Geometry check sheet. Reference: the model listing, model coordinates, mm. A direction names the side the tool comes from. Round coordinates to 2 decimals unless told otherwise and drop trailing zeros. Write each loop counter-clockwise with the first axis right and the second up, starting at its lowest first coordinate (ties: lowest second). Pieces come first, ordered by that corner, then holes.
Item 1: Cross-section at C-C (z = 4.5). Enter the section's corners in (x, y).
Item 2: Cross-section at D-D (x = -0.25). Enter the section's corners in (y, z), then the cut area to 3 significant figures.
Item 3: Depth check by flat-ended pin: P1, Ø0.6, axis at x = 5, z = 1.5, coming from the -Y side; P2, Ø0.8, axis at y = 0.5, z = -3, coming from the +X side; P3, Ø3.5, axis at x = 10.1, z = -1.5, coming from the +Y side. Enter the tip coordinate at first touch or a pass-through.
Item 4: Draft check along Y on faces 1 (the face through (2.2, 4.2, 3.5)), 2 (the face through (5.754, -5.325, 1.728)), 3 (the face through (10, 3.5, 2)), 4 (the face through (4.5, 2.6, 0.8)). Enter one of: pulls with the +Y half, pulls with the -Y half, needs draft (parallel to the pull), parting line crosses it, or undercut.
Item 5: Cross-section at A-A (z = -1.5). Enter the section's corners in (x, y), then the cut area to 3 significant figures.
Item 6: Cross-section at B-B (z = 10.25). Enter the section's corners in (x, y).
Item 7: Access from +Z, -Z, +X, -X, +Y, -Y to the whole of each face (thin tool, end or side, straight path). Record for faces 5 (the face through (0, 0, 0)), 6 (the face through (6.81, 4.49, -0.13)), 7 (the face through (7.6, 3, 0)), 8 (the face through (10, 4, 2)), 9 (the face through (-4, 1, 3.5)).
Item 8: Scan lines: probe 1 along X at (y, z) = (3.75, -1.5); probe 2 along X at (y, z) = (3.95, 4.5); probe 3 along Y at (x, z) = (5.8, 1.5). Record each from-to range of solid material in increasing order.
from build123d import *

# Parameters (mm, degrees)
SKETCH1_W            = 9
SKETCH1_H            = 7
BOSS_EXTRUDE1_DEPTH  = 7
SKETCH4_W            = 0.725
SKETCH4_H            = 0.725
BOSS_EXTRUDE3_DEPTH  = 0.3
SKETCH7_W            = 6.8
SKETCH7_H            = 1
BOSS_EXTRUDE5_DEPTH  = 1
FILLET1_R            = 0.5
SKETCH8_W            = 15.5
SKETCH8_H            = 14
BOSS_EXTRUDE6_DEPTH  = 0.5
EXTRUDE_9_DEPTH      = 10
EXTRUDE_9_DEPTH_BACK = 2.1
SKETCH_6_R           = 1
SKETCH10_W           = 10.53
SKETCH10_H           = 0.5
BOSS_EXTRUDE9_DEPTH  = 5
SKETCH_3_R           = 1.05
CUT_EXTRUDE_2_DEPTH  = 0.5
SKETCH_5_R           = 3.25
EXTRUDE_2_DEPTH      = 20.5
SKETCH_7_R           = 1.05
CUT_EXTRUDE_3_DEPTH  = 1.6


with BuildPart() as part:
    # Sketch1 → Boss-Extrude1 (new body)
    with BuildSketch(Plane(origin=(0, 0, 0), x_dir=(1, 0, 0), z_dir=(0, 1, 0))):
        Rectangle(SKETCH1_W, SKETCH1_H)
    extrude(amount=BOSS_EXTRUDE1_DEPTH)

    # Sketch4 → Boss-Extrude3 (add)
    with BuildSketch(Plane(origin=(4.5, 0, 0), x_dir=(0, 0, -1), z_dir=(1, 0, 0))):
        with Locations((-3.1375, 6.6375)):
            Rectangle(SKETCH4_W, SKETCH4_H)
        with Locations((3.1375, 6.6375)):
            Rectangle(SKETCH4_W, SKETCH4_H)
        with Locations((-3.1375, 0.3625)):
            Rectangle(SKETCH4_W, SKETCH4_H)
        with Locations((3.1375, 0.3625)):
            Rectangle(SKETCH4_W, SKETCH4_H)
    extrude(amount=BOSS_EXTRUDE3_DEPTH)

    # Sketch7 → Boss-Extrude5 (add)
    with BuildSketch(Plane(origin=(4.5, 0, 0), x_dir=(0, 0, -1), z_dir=(1, 0, 0))):
        with Locations((0, 0.6)):
            Rectangle(SKETCH7_W, SKETCH7_H)
        with Locations((0, 6.4)):
            Rectangle(SKETCH7_W, SKETCH7_H)
    extrude(amount=BOSS_EXTRUDE5_DEPTH)

    # Fillet1
    # the kernel refuses this fillet: 0.5 mm, written as the material it adds along each edge
    with BuildSketch(Plane(origin=(4.5, 6.9, 3.525), x_dir=(0, 1, 0), z_dir=(0, 0, -1))) as fillet1_piece_1_section:
        with BuildLine():
            CenterArc((0.5, 0.3), FILLET1_R, 180, 36.869897646)
            Line((0, 0.3), (0, 0))
            Line((0, 0), (0.1, 0))
        make_face()
    fillet1_piece_1 = extrude(amount=7.05, mode=Mode.PRIVATE)
    fillet1_piece_1 = split(fillet1_piece_1, bisect_by=Plane(origin=(4.5, 6.9, -3.4), z_dir=(0, 0, 1)), keep=Keep.TOP, mode=Mode.PRIVATE)
    fillet1_piece_1 = split(fillet1_piece_1, bisect_by=Plane(origin=(4.5, 6.9, 3.4), z_dir=(0, 0, -1)), keep=Keep.TOP, mode=Mode.PRIVATE)
    add(fillet1_piece_1)
    with BuildSketch(Plane(origin=(4.5, 5.9, 3.4), x_dir=(0, 0, 1), z_dir=(0, 1, 0))) as fillet1_piece_2:
        with BuildLine():
            CenterArc((0.5, 0.3), FILLET1_R, 180, 36.869897646)
            Line((0, 0.3), (0, 0))
            Line((0, 0), (0.1, 0))
        make_face()
    extrude(amount=0.375)
    with BuildSketch(Plane(origin=(4.5, 5.9, -3.4), x_dir=(0, -1, 0), z_dir=(0, 0, 1)), Plane(origin=(4.5, 1.1, 3.4), x_dir=(0, 1, 0), z_dir=(0, 0, -1))) as fillet1_piece_3:
        with BuildLine():
            CenterArc((FILLET1_R, FILLET1_R), FILLET1_R, 180, 90)
            Line((0, FILLET1_R), (0, 0))
            Line((0, 0), (FILLET1_R, 0))
        make_face()
    extrude(amount=6.8)
    with BuildSketch(Plane(origin=(4.5, 7.025, -3.4), x_dir=(0, 0, -1), z_dir=(0, -1, 0))) as fillet1_piece_4_section:
        with BuildLine():
            CenterArc((0.5, 0.3), FILLET1_R, 180, 36.869897646)
            Line((0, 0.3), (0, 0))
            Line((0, 0), (0.1, 0))
        make_face()
    fillet1_piece_4 = extrude(amount=1.125, mode=Mode.PRIVATE)
    fillet1_piece_4 = split(fillet1_piece_4, bisect_by=Plane(origin=(4.5, 6.9, -3.4), z_dir=(0, -1, 0)), keep=Keep.TOP, mode=Mode.PRIVATE)
    add(fillet1_piece_4)
    with BuildSketch(Plane(origin=(4.5, 1.1, -3.4), x_dir=(0, 0, -1), z_dir=(0, -1, 0))) as fillet1_piece_5_section:
        with BuildLine():
            CenterArc((0.5, 0.3), FILLET1_R, 180, 36.869897646)
            Line((0, 0.3), (0, 0))
            Line((0, 0), (0.1, 0))
        make_face()
    fillet1_piece_5 = extrude(amount=1.125, mode=Mode.PRIVATE)
    fillet1_piece_5 = split(fillet1_piece_5, bisect_by=Plane(origin=(4.5, 0.1, -3.4), z_dir=(0, 1, 0)), keep=Keep.TOP, mode=Mode.PRIVATE)
    add(fillet1_piece_5)
    with BuildSketch(Plane(origin=(4.5, -0.025, 3.4), x_dir=(0, 0, 1), z_dir=(0, 1, 0))) as fillet1_piece_6_section:
        with BuildLine():
            CenterArc((0.5, 0.3), FILLET1_R, 180, 36.869897646)
            Line((0, 0.3), (0, 0))
            Line((0, 0), (0.1, 0))
        make_face()
    fillet1_piece_6 = extrude(amount=1.125, mode=Mode.PRIVATE)
    fillet1_piece_6 = split(fillet1_piece_6, bisect_by=Plane(origin=(4.5, 0.1, 3.4), z_dir=(0, 1, 0)), keep=Keep.TOP, mode=Mode.PRIVATE)
    add(fillet1_piece_6)
    with BuildSketch(Plane(origin=(4.5, 0.1, -2.775), x_dir=(1, 0, 0), z_dir=(0, 0, 1))) as fillet1_piece_7:
        with BuildLine():
            CenterArc((0.3, -0.5), FILLET1_R, 90, 36.869897646)
            Line((0, -0.1), (0, 0))
            Line((0, 0), (0.3, 0))
        make_face()
    extrude(amount=5.55)
    with BuildSketch(Plane(origin=(4.5, 5.15, 3.4), x_dir=(0, 0, 1), z_dir=(0, 1, 0))) as fillet1_piece_8a_section:
        with BuildLine():
            CenterArc((0.5, 0.3), FILLET1_R, 180, 36.869897646)
            Line((0, 0.3), (0, 0))
            Line((0, 0), (0.1, 0))
        make_face()
    fillet1_piece_8a = extrude(amount=1.125, mode=Mode.PRIVATE)
    fillet1_piece_8a = split(fillet1_piece_8a, bisect_by=Plane(origin=(4.5, 5.9, 3.4), z_dir=(0, -1, 0)), keep=Keep.TOP, mode=Mode.PRIVATE)
    with BuildSketch(Plane(origin=(4.5, 5.9, -3.4), x_dir=(0, -1, 0), z_dir=(0, 0, 1))) as fillet1_piece_8b_section:
        with BuildLine():
            CenterArc((FILLET1_R, FILLET1_R), FILLET1_R, 180, 90)
            Line((0, FILLET1_R), (0, 0))
            Line((0, 0), (FILLET1_R, 0))
        make_face()
    fillet1_piece_8b = extrude(amount=8.05, mode=Mode.PRIVATE)
    fillet1_piece_8b = split(fillet1_piece_8b, bisect_by=Plane(origin=(4.5, 5.9, 3.5), z_dir=(0, 0, -1)), keep=Keep.TOP, mode=Mode.PRIVATE)
    fillet1_piece_8b = split(fillet1_piece_8b, bisect_by=Plane(origin=(4.5, 5.9, 3.4), z_dir=(0, 0, 1)), keep=Keep.TOP, mode=Mode.PRIVATE)
    fillet1_piece_8 = fillet1_piece_8a & fillet1_piece_8b
    add(fillet1_piece_8)
    with BuildSketch(Plane(origin=(4.5, 5.9, -4.65), x_dir=(0, -1, 0), z_dir=(0, 0, 1))) as fillet1_piece_9a_section:
        with BuildLine():
            CenterArc((FILLET1_R, FILLET1_R), FILLET1_R, 180, 90)
            Line((0, FILLET1_R), (0, 0))
            Line((0, 0), (FILLET1_R, 0))
        make_face()
    fillet1_piece_9a = extrude(amount=8.05, mode=Mode.PRIVATE)
    fillet1_piece_9a = split(fillet1_piece_9a, bisect_by=Plane(origin=(4.5, 5.9, -3.5), z_dir=(0, 0, 1)), keep=Keep.TOP, mode=Mode.PRIVATE)
    fillet1_piece_9a = split(fillet1_piece_9a, bisect_by=Plane(origin=(4.5, 5.9, -3.4), z_dir=(0, 0, -1)), keep=Keep.TOP, mode=Mode.PRIVATE)
    with BuildSketch(Plane(origin=(4.5, 6.275, -3.4), x_dir=(0, 0, -1), z_dir=(0, -1, 0))) as fillet1_piece_9b_section:
        with BuildLine():
            CenterArc((0.5, 0.3), FILLET1_R, 180, 36.869897646)
            Line((0, 0.3), (0, 0))
            Line((0, 0), (0.1, 0))
        make_face()
    fillet1_piece_9b = extrude(amount=1.125, mode=Mode.PRIVATE)
    fillet1_piece_9b = split(fillet1_piece_9b, bisect_by=Plane(origin=(4.5, 5.9, -3.4), z_dir=(0, -1, 0)), keep=Keep.TOP, mode=Mode.PRIVATE)
    fillet1_piece_9 = fillet1_piece_9a & fillet1_piece_9b
    add(fillet1_piece_9)
    with BuildSketch(Plane(origin=(4.5, 1.85, -3.4), x_dir=(0, 0, -1), z_dir=(0, -1, 0))) as fillet1_piece_10a_section:
        with BuildLine():
            CenterArc((0.5, 0.3), FILLET1_R, 180, 36.869897646)
            Line((0, 0.3), (0, 0))
            Line((0, 0), (0.1, 0))
        make_face()
    fillet1_piece_10a = extrude(amount=1.125, mode=Mode.PRIVATE)
    fillet1_piece_10a = split(fillet1_piece_10a, bisect_by=Plane(origin=(4.5, 1.1, -3.4), z_dir=(0, 1, 0)), keep=Keep.TOP, mode=Mode.PRIVATE)
    with BuildSketch(Plane(origin=(4.5, 1.1, 3.4), x_dir=(0, 1, 0), z_dir=(0, 0, -1))) as fillet1_piece_10b_section:
        with BuildLine():
            CenterArc((FILLET1_R, FILLET1_R), FILLET1_R, 180, 90)
            Line((0, FILLET1_R), (0, 0))
            Line((0, 0), (FILLET1_R, 0))
        make_face()
    fillet1_piece_10b = extrude(amount=8.05, mode=Mode.PRIVATE)
    fillet1_piece_10b = split(fillet1_piece_10b, bisect_by=Plane(origin=(4.5, 1.1, -3.5), z_dir=(0, 0, 1)), keep=Keep.TOP, mode=Mode.PRIVATE)
    fillet1_piece_10b = split(fillet1_piece_10b, bisect_by=Plane(origin=(4.5, 1.1, -3.4), z_dir=(0, 0, -1)), keep=Keep.TOP, mode=Mode.PRIVATE)
    fillet1_piece_10 = fillet1_piece_10a & fillet1_piece_10b
    add(fillet1_piece_10)
    with BuildSketch(Plane(origin=(4.5, 1.1, 4.65), x_dir=(0, 1, 0), z_dir=(0, 0, -1))) as fillet1_piece_11a_section:
        with BuildLine():
            CenterArc((FILLET1_R, FILLET1_R), FILLET1_R, 180, 90)
            Line((0, FILLET1_R), (0, 0))
            Line((0, 0), (FILLET1_R, 0))
        make_face()
    fillet1_piece_11a = extrude(amount=8.05, mode=Mode.PRIVATE)
    fillet1_piece_11a = split(fillet1_piece_11a, bisect_by=Plane(origin=(4.5, 1.1, 3.5), z_dir=(0, 0, -1)), keep=Keep.TOP, mode=Mode.PRIVATE)
    fillet1_piece_11a = split(fillet1_piece_11a, bisect_by=Plane(origin=(4.5, 1.1, 3.4), z_dir=(0, 0, 1)), keep=Keep.TOP, mode=Mode.PRIVATE)
    with BuildSketch(Plane(origin=(4.5, 0.725, 3.4), x_dir=(0, 0, 1), z_dir=(0, 1, 0))) as fillet1_piece_11b_section:
        with BuildLine():
            CenterArc((0.5, 0.3), FILLET1_R, 180, 36.869897646)
            Line((0, 0.3), (0, 0))
            Line((0, 0), (0.1, 0))
        make_face()
    fillet1_piece_11b = extrude(amount=1.125, mode=Mode.PRIVATE)
    fillet1_piece_11b = split(fillet1_piece_11b, bisect_by=Plane(origin=(4.5, 1.1, 3.4), z_dir=(0, 1, 0)), keep=Keep.TOP, mode=Mode.PRIVATE)
    fillet1_piece_11 = fillet1_piece_11a & fillet1_piece_11b
    add(fillet1_piece_11)

    # Sketch8 → Boss-Extrude6 (add)
    with BuildSketch(Plane(origin=(5.5, 0, 0), x_dir=(0, 0, -1), z_dir=(1, 0, 0))):
        with Locations((-4.25, 0)):
            Rectangle(SKETCH8_W, SKETCH8_H)
    extrude(amount=BOSS_EXTRUDE6_DEPTH)

    # ｽｹｯﾁ6 → ﾎﾞｽ - 押し出し9 (add, two sides: drawn at the far end of the back side and taken through both)
    with BuildSketch(Plane.ZY.offset(-5.5).offset(-EXTRUDE_9_DEPTH_BACK)):
        with Locations((0, 3.5)):
            Circle(SKETCH_6_R)
    extrude(amount=EXTRUDE_9_DEPTH + EXTRUDE_9_DEPTH_BACK)

    # Sketch10 → Boss-Extrude9 (add)
    with BuildSketch(Plane(origin=(7.6, 0, 0), x_dir=(0, 0, -1), z_dir=(1, 0, 0))):
        with Locations((-1.765, 3.75)):
            Rectangle(SKETCH10_W, SKETCH10_H)
    extrude(amount=BOSS_EXTRUDE9_DEPTH)

    # ｽｹｯﾁ3 → ｶｯﾄ - 押し出し2 (cut)
    with BuildSketch(Plane(origin=(6, 0, 0), x_dir=(0, 0, -1), z_dir=(1, 0, 0))):
        with Locations((-1.5, -4.3)):
            Circle(SKETCH_3_R)
        with Locations((-7.5, -4.3)):
            Circle(SKETCH_3_R)
    extrude(amount=-CUT_EXTRUDE_2_DEPTH, mode=Mode.SUBTRACT)

    # ｽｹｯﾁ5 → ﾎﾞｽ - 押し出し2 (add)
    with BuildSketch(Plane.XY.offset(3.5)):
        with Locations(Location((-1.25, 3.25, 0), (0, 0, 180))):
            Circle(SKETCH_5_R)
    extrude(amount=EXTRUDE_2_DEPTH)

    # ｽｹｯﾁ7 → ｶｯﾄ - 押し出し3 (cut)
    with BuildSketch(Plane(origin=(0, 3.5, 0), x_dir=(-1, 0, 0), z_dir=(0, -1, 0))):
        with Locations(Location((-10.1, -4.5, 0), (0, 0, 90))):
            Circle(SKETCH_7_R)
        with Locations(Location((-10.1, 1.5, 0), (0, 0, 90))):
            Circle(SKETCH_7_R)
    extrude(amount=-CUT_EXTRUDE_3_DEPTH, mode=Mode.SUBTRACT)


solid = part.part
Resolved:
1. outline: circle Ø6.5 at (-1.25, 3.25); (5.5, -7) - (6, -7) - (6, 7) - (5.5, 7) - close; (7.6, 3.5) - (9.05, 3.5) - (9.05, 4) - (7.6, 4) - close; (11.15, 3.5) - (12.6, 3.5) - (12.6, 4) - (11.15, 4) - close
2. outline: (0, -3.5) - (7, -3.5) - (7, 3.5) - (6.34, 3.5) - (6.34, 24) - (0.16, 24) - (0.16, 3.5) - (0, 3.5) - close
2. area: 176 mm2
3. P1: stops at y = 0.09
3. P2: stops at x = 6
3. P3: stops at y = 4
4. face 1: needs draft
4. face 2: undercut
4. face 3: pulls with the -Y half
4. face 4: undercut
5. outline: (-4.5, 0) - (4.5, 0) arc R0.5 cw to (4.8, 0.1) - (5.5, 0.1) - (5.5, -7) - (6, -7) - (6, 7) - (5.5, 7) - (5.5, 6.9) - (4.8, 6.9) arc R0.5 cw to (4.5, 7) - (-4.5, 7) - close; (7.6, 3.5) - (9.05, 3.5) - (9.05, 4) - (7.6, 4) - close; (11.15, 3.5) - (12.6, 3.5) - (12.6, 4) - (11.15, 4) - close; hole (4.5, 1.6) arc R0.5 ccw to (5, 1.1) - (5.5, 1.1) - (5.5, 5.9) - (5, 5.9) arc R0.5 ccw to (4.5, 5.4) - close
5. area: 73.6 mm2
6. outline: circle Ø6.5 at (-1.25, 3.25); (5.5, -7) - (6, -7) - (6, 7) - (5.5, 7) - close
7. face 5: +Z, -Z, -X, -Y
7. face 6: none
7. face 7: +Z, -Z, +X, -Y
7. face 8: +Z, -Z, +X, +Y
7. face 9: +Z, -X, -Y
8. probe 1: x = -4.5 to 4.5, 5.5 to 6, 7.6 to 9.05, 11.15 to 12.6
8. probe 2: x = -4.42 to 1.92, 5.5 to 6, 7.6 to 9.05, 11.15 to 12.6
8. probe 3: y = -7 to -5.35, -3.25 to 7
